Input: dimensioned drawing with shaded views. Units: mm. Origin: part minimum x, y, z. A direction names the side the tool comes from. Give positions to 0.01 mm unless a question says otherwise; leave off trailing zeros. Write each loop counter-clockwise with the first axis right and the second up, starting at its lowest first coordinate (ties: lowest second). Pieces come first, ordered by that corner, then holes. Notation, with made-up numbers: (-30.5, 54) - (17.5, 54) arc R34 cw to (17.5, 90) - close; hole circle Ø11 at (-11, 63.25). An arc over 180 degrees is marked (long way). Answer as CSV lines item,"result".
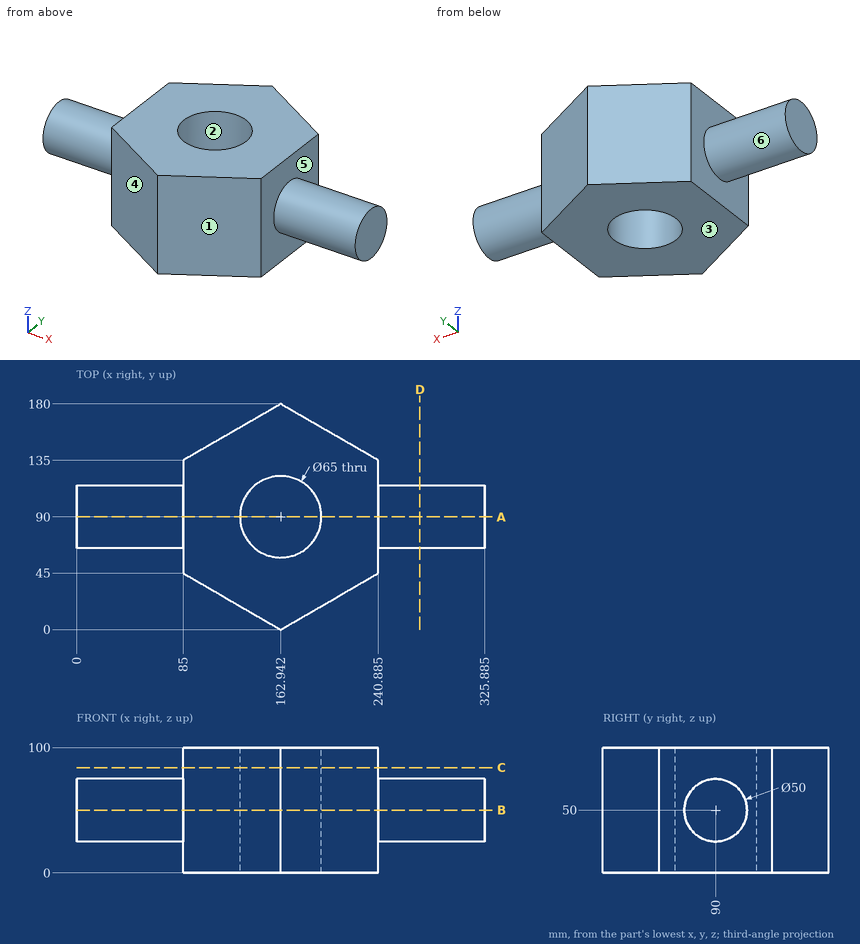
Item 1: Contact query for flat-ended pins moving along their axis: pin 1 (6 mm diameter, centred on y = 96.5, z = 39, fed in from -X); pin 2 (10 mm diameter, centred on x = 67, y = 80, fed in from -Z) (1 decimal); pin 3 (12 mm diameter, centred on x = 53, y = 106.5, fed in from +Z); pin 4 (1.5 mm diameter, centred on y = 100.5, z = 75.5, fed in from +X) (1 decimal). Output: stop coordinate, or through.
The answers:
pin 1,"x = 0"
pin 2,"z = 25.5"
pin 3,"z = 72.69"
pin 4,"x = 240.9"
Item 2: Cut plane B-B on z = 50. Return the cut outline in (x, y) (1 decimal), plus the area to 3 significant figures.
The answers:
outline,"(0, 65) - (85, 65) - (85, 45) - (162.9, 0) - (240.9, 45) - (240.9, 65) - (325.9, 65) - (325.9, 115) - (240.9, 115) - (240.9, 135) - (162.9, 180) - (85, 135) - (85, 115) - (0, 115) - close; hole circle Ø65 at (162.9, 90)"
area,"26,200 mm²"
Item 3: Cut plane C-C on z = 84. Return the cut outline in (x, y) (1 decimal).
The answers:
outline,"(85, 45) - (162.9, 0) - (240.9, 45) - (240.9, 135) - (162.9, 180) - (85, 135) - close; hole circle Ø65 at (162.9, 90)"
Item 4: Mould query, pull axis Y, two halves, no side actions, for the marked faces 1, 2 and 3. Classes: +Y half, -Y half, draft (parallel to the pull), parting line (faces both ways), or undercut.
The answers:
face 1,"-Y half"
face 2,"undercut"
face 3,"draft"
Item 5: Cut plane A-A on y = 90. Return the cut outline in (x, z) (1 decimal).
The answers:
outline,"(0, 25) - (85, 25) - (85, 0) - (130.4, 0) - (130.4, 100) - (85, 100) - (85, 75) - (0, 75) - close; (195.4, 0) - (240.9, 0) - (240.9, 25) - (325.9, 25) - (325.9, 75) - (240.9, 75) - (240.9, 100) - (195.4, 100) - close"
Item 6: Ray query, line 1 (X direction, y = 57, z = 10) (1 decimal); line 2 (Y direction, x = 162, z = 45.5) (1 decimal); line 3 (Y direction, x = 167, z = 10.5) (1 decimal). Return the intervals inside material, ascending. Write a range as from..to.
The answers:
line 1,"85..240.9"
line 2,"0.5..57.5, 122.5..179.5"
line 3,"2.3..57.8, 122.2..177.7"
Item 7: Cut plane D-D on x = 274. Return the cut outline in (y, z).
The answers:
outline,"circle Ø50 at (90, 50)"
Item 8: Reachability of the marked faces 4, 5 and 6 from +Z, -Z, +X, -X, +Y, -Y: full face, straight path, thin tool, end or side. Return the list, or none.
The answers:
face 4,"+Z, -Z, -X, -Y"
face 5,"+X"
face 6,"-X"
